Work out the finished part from the listing and answer in its coordinate system (mm). Give positions to 0.01 mm unless a question says otherwise; leave off trailing zeros. Write each loop counter-clockwise with the first axis right and the second up, starting at its lowest first coordinate (ties: lowest second). Pieces come first, ordered by that corner, then holes.
1) Straight lines are drawn through the part: probe 1 along Z at (x, y) = (-27, 0.8); probe 2 along Z at (x, y) = (-0.5, 0.9); probe 3 along X at (y, z) = (0.55, 41). For each, find the intervals that lie inside material, in ascending order.
2) Determine the mould class of faces 1 (the face through (-28.895, 0.783, -8.305)), 2 (the face through (-3.358, 0.783, -0.981)), 3 (the face through (-17, 1, -2.792)) for opening direction X: pulls with the +X half, pulls with the -X half, needs draft (parallel to the pull), parting line crosses it, or undercut.
3) Find section D-D (z = 11). Determine the outline of the cut face in (x, y), plus the area to 3 significant figures.
4) Find section C-C (x = 23). Determine the outline of the cut face in (y, z).
5) Find section A-A (x = -6). Determine the outline of the cut face in (y, z), plus the area to 3 significant figures.
6) Find section B-B (y = 0.65). Count the separate pieces of the cut face and the enclosed holes in it, plus the area to 3 significant figures.
7) Given pin 1 Ø0.8 at (x, y) = (-16, 1) entering from +Z; pin 2 Ø0.8 at (y, z) = (0.5, 16) entering from -X, each flat-ended and moving along its own axis, determine where each tip first touches the part or whether it passes through.
Autodesk Inventor part; units mm, degrees
ref_plane "YZ Plane" through (0, 0, 0) normal (1, 0, 0) x (0, 1, 0)
ref_plane "XZ Plane" through (0, 0, 0) normal (0, 1, 0) x (-1, 0, 0)
ref_plane "XY Plane" through (0, 0, 0) normal (0, 0, 1) x (1, 0, 0)
sketch "Sketch1" plane through (0, 0, 0) normal (0, 1, 0) x (-1, 0, 0)
  circle A0 centre (1.4772, 41.6579) radius 2.1844
  circle A1 centre (26.8772, 41.6579) radius 2.1844
  circle A2 centre (26.8772, -9.1421) radius 2.1844
  circle A3 centre (1.4772, -9.1421) radius 2.1844
  arc A4 (1.4487, 47.8916) -> (-3.6864, 45.1505) centre (1.4772, 41.6579) ccw
  arc A5 (26.8481, 35.3079) -> (26.8191, 48.0076) centre (26.8772, 41.6579) ccw
  arc A6 (26.8487, -15.4921) -> (26.8487, -2.7922) centre (26.8772, -9.1421) ccw
  circle A7 centre (-23.9228, 6.7329) radius 2.0955
  arc A8 (-27.8677, 9.4012) -> (-26.6575, 2.8337) centre (-23.9228, 6.7329) ccw
  line L0 (-3.6864, 45.1505) -> (-27.8677, 9.4012)
  line L1 (-26.6575, 2.8337) -> (-2.169, -14.341)
  line L2 (26.8772, 48.0079) -> (1.4487, 47.8916)
  line L3 (26.8481, 35.3079) -> (7.8277, 35.3949)
  line L4 (1.4487, 29.045) -> (1.4487, 3.5578)
  line L5 (26.9057, -2.7922) -> (7.7987, -2.7922)
  line L6 (26.9057, -15.4921) -> (1.4487, -15.4921)
  arc A9 (1.5057, -2.7922) -> (1.4487, -2.7922) centre (1.4772, -9.1421) ccw
  arc A10 (-2.169, -14.341) -> (1.5057, -15.4921) centre (1.4772, -9.1421) ccw
  arc A11 (7.8277, 35.3949) -> (1.4487, 29.045) centre (7.7987, 29.045) ccw
  arc A12 (1.4487, 3.5578) -> (7.7987, -2.7922) centre (7.7987, 3.5578) ccw
  point P0 (0, 0)
  dimension "d0" = 4.191
  dimension "d1" = 9.525
  dimension "d2" = 25.4
  dimension "d3" = 6.35
extrude "Extrusion1" add sketch "Sketch1" along normal blind 1.5875
properties part number "gusset" material "Acetal Resin, White"
Results:
1. probe 1: z = -15.49 to -11.32, -6.96 to -2.79, 35.31 to 39.48, 43.84 to 48.01
1. probe 2: z = -15.42 to -11.1, -7.19 to 39.7, 43.61 to 47.81
1. probe 3: x = -33.19 to -28.96, -24.79 to -3.56, 0.61 to 6.49
2. face 1: undercut
2. face 2: pulls with the -X half
2. face 3: needs draft
3. outline: (-1.45, 0) - (26.79, 0) - (26.79, 1.59) - (-1.45, 1.59) - close
3. area: 44.8 mm2
4. outline: (0, 0.27) - (1.59, 0.27) - (1.59, 4.85) - (0, 4.85) - close; (0, 8.61) - (1.59, 8.61) - (1.59, 16.6) - (0, 16.6) - close
5. outline: (0, -15.49) - (1.59, -15.49) - (1.59, -2.53) - (0, -2.53) - close; (0, 35.13) - (1.59, 35.13) - (1.59, 47.91) - (0, 47.91) - close
5. area: 40.9 mm2
6. separate pieces: 1
6. enclosed holes: 5
6. area: 1,810 mm2
7. pin 1: stops at z = 47.96
7. pin 2: stops at x = -1.45
